The model under review builds one solid part; all positions refer to its coordinate system, in mm. Round coordinates to 2 decimals unless told otherwise and drop trailing zeros. Order: outer loops, then holes, each group sorted by start corner. A loop starts at its lowest first (then second) coordinate and runs counter-clockwise, first axis right, second up.
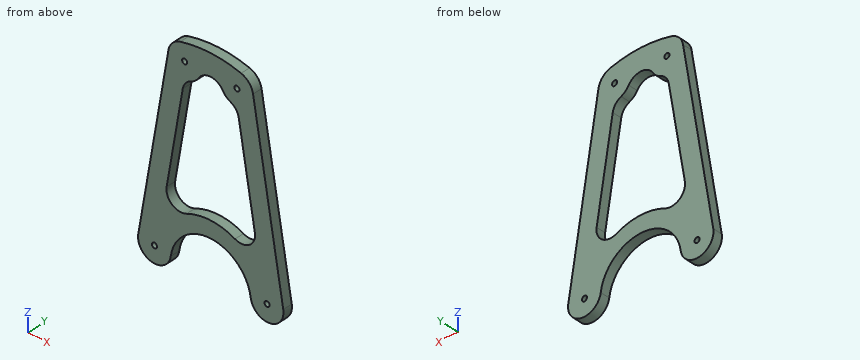
Autodesk Inventor part; units mm, degrees
ref_plane "YZ Plane" through (0, 0, 0) normal (1, 0, 0) x (0, 1, 0)
ref_plane "XZ Plane" through (0, 0, 0) normal (0, 1, 0) x (-1, 0, 0)
ref_plane "XY Plane" through (0, 0, 0) normal (0, 0, 1) x (1, 0, 0)
sketch "Sketch1" plane through (0, 0, 0) normal (0, 1, 0) x (-1, 0, 0)
  circle A0 centre (0, 0) radius 38.1 construction
  line L0 (38.1, 0) -> (-38.1, 0) construction
  circle A1 centre (38.1, 0) radius 1.7526
  circle A2 centre (-38.1, 0) radius 1.7526
  circle A3 centre (38.1, 0) radius 7.9375 construction
  circle A4 centre (-38.1, 0) radius 7.9375 construction
  line L1 (0, 0) -> (0, -38.1) construction
  circle A5 centre (0, 56.6406) radius 76.2 construction
  circle A6 centre (-17.6676, 122.5771) radius 7.9375 construction
  circle A7 centre (-17.6676, 122.5771) radius 1.7526
  circle A8 centre (-38.1, 0) radius 11.1125
  circle A9 centre (38.1, 0) radius 11.1125
  circle A10 centre (-17.6676, 122.5771) radius 11.1125
  line L2 (0, 56.6406) -> (0, 132.8406) construction
  line L3 (0, 56.6406) -> (-17.6676, 122.5771) construction
  line L4 (-49.0613, 1.8271) -> (-28.6289, 124.4043)
  line L5 (-38.1, 0) -> (-17.6676, 122.5771) construction
  circle A11 centre (17.6676, 122.5771) radius 7.9375 construction
  circle A12 centre (17.6676, 122.5771) radius 1.7526
  circle A13 centre (17.6676, 122.5771) radius 11.1125
  line L6 (49.0613, 1.8271) -> (28.6289, 124.4043)
  line L7 (38.1, 0) -> (17.6676, 122.5771) construction
  arc A14 (20.5438, 133.311) -> (-20.5438, 133.311) centre (0, 56.6406) ccw
  arc A15 (-44.3023, -9.2206) -> (44.3023, -9.2206) centre (0, 56.6406) ccw
  arc A16 (17.6676, 122.5771) -> (-17.6676, 122.5771) centre (0, 56.6406) ccw
  arc A17 (-38.1, 0) -> (38.1, 0) centre (0, 56.6406) ccw
  line L8 (-34.7257, 10.5878) -> (-17.9101, 111.4673)
  line L9 (34.7257, 10.5878) -> (17.9101, 111.4673)
  circle A18 centre (0, 0) radius 19.5594
  arc A19 (27.0858, -1.4751) -> (-27.0858, -1.4751) centre (0, -5.1027) ccw
  circle A20 centre (0, 0) radius 22.225 construction
  arc A21 (38.1, 0) -> (-38.1, 0) centre (0, -5.1027) ccw
  point P0 (49.0613, 1.8271)
  point P1 (6.7353, 124.57)
  point P2 (17.9101, 111.4673)
  point P3 (28.4052, -5.4312)
  point P4 (-28.4052, -5.4312)
  point P5 (-6.7353, 124.57)
  point P6 (17.1322, -9.437)
  point P7 (-17.1322, -9.437)
  point P8 (34.5232, 11.8029)
  point P9 (-34.5232, 11.8029)
  dimension "d5" = 152.4
  dimension "d0" = 76.2
  dimension "d1" = 3.5052
  dimension "d2" = 3.5052
  dimension "d3" = 15.875
  dimension "d4" = 15.875
  dimension "d8" = 15.875
  dimension "d9" = 3.5052
  dimension "d11" = 15
  dimension "d12" = 79.375
  dimension "d13" = 79.375
  dimension "d17" = 11.1125
  dimension "d18" = 11.1125
  dimension "d20" = 12.7
  dimension "d21" = 44.45
  dimension "d22" = 11.1125
extrude "Extrusion1" add sketch "Sketch1" along normal blind 6.35 contours A1 A21 A9 A17 | A1 A17 A9 A21 | A21 L9 A13 L6 A9 | A9 L9 A21 | A9 A19 A8 L8 A21 L9 | A13 | A21 A8 L4 A10 L8 | L8 A8 A21 | A8 A17 A2 A21 | A8 A21 A2 A17 | A13 A16 A10 A14 | A10
fillet "Fillet1" radius 9.525 6 edges at (17.9101, 3.175, 111.4673) (6.7353, 3.175, 124.57) (-6.7353, 3.175, 124.57) (-17.9101, 3.175, 111.4673) (-34.5232, 3.175, 11.8029) (34.5232, 3.175, 11.8029)
equation "\"d1\" = d2"
equation "\"d9\" = d2"
equation "\"d13\" = d12"
properties part number "Upright - Lower" material "Aluminum 6061"
(1) We need section D-D (y = 1.25). Count the separate pieces of the cut face and the enclosed holes in it, and give its area (3 significant figures).
(2) We need section A-A (x = -38.1). Give the boundary of the cut face in (y, z), and give its area (3 significant figures).
(3) We need section C-C (z = 78). Give the boundary of the cut face in (x, y), and give its area (3 significant figures).
(4) We need section B-B (z = 0). Give the boundary of the cut face in (x, y), and give its area (3 significant figures).
(5) Clearance check with a flat-ended pin moving along its axis: P1, Ø2, axis at x = 38.1, z = 0, coming from the +Y side. State where the tip first meets the part, or that it passes through.
(6) To check wall thickness, follow L1, parallel to X at y = 2.75, z = 0; L2, parallel to X at y = 2, z = 85.5; L3, parallel to X at y = 5, z = 80.5. State the ranges of each line that lie inside material, in increasing order.
Verdict:
1. separate pieces: 1
1. enclosed holes: 5
1. area: 5,610 mm2
2. outline: (0, -11.11) - (6.35, -11.11) - (6.35, -1.75) - (0, -1.75) - close; (0, 1.75) - (6.35, 1.75) - (6.35, 67.59) - (0, 67.59) - close
2. area: 477 mm2
3. outline: (-36.36, 0) - (-23.49, 0) - (-23.49, 6.35) - (-36.36, 6.35) - close; (23.49, 0) - (36.36, 0) - (36.36, 6.35) - (23.49, 6.35) - close
3. area: 164 mm2
4. outline: (-49.21, 0) - (-39.85, 0) - (-39.85, 6.35) - (-49.21, 6.35) - close; (-36.35, 0) - (-26.85, 0) - (-26.85, 6.35) - (-36.35, 6.35) - close; (26.85, 0) - (36.35, 0) - (36.35, 6.35) - (26.85, 6.35) - close; (39.85, 0) - (49.21, 0) - (49.21, 6.35) - (39.85, 6.35) - close
4. area: 240 mm2
5. P1: passes through
6. L1: x = -49.21 to -39.85, -36.35 to -26.85, 26.85 to 36.35, 39.85 to 49.21
6. L2: x = -35.11 to -22.24, 22.24 to 35.11
6. L3: x = -35.95 to -23.07, 23.07 to 35.95
